Autodesk Inventor part; units mm, degrees
ref_plane "YZ Plane" through (0, 0, 0) normal (1, 0, 0) x (0, 1, 0)
ref_plane "XZ Plane" through (0, 0, 0) normal (0, 1, 0) x (-1, 0, 0)
ref_plane "XY Plane" through (0, 0, 0) normal (0, 0, 1) x (1, 0, 0)
sketch "Sketch15" plane through (0, 0, 0) normal (0, 0, 1) x (1, 0, 0)
  line L0 (0, 0) -> (0, 1.4)
  line L1 (0.2309, 1.8) -> (1.5, 1.8)
  line L2 (1.5, 1.8) -> (1.5, 2)
  line L3 (1.5, 2) -> (1.7, 2)
  line L4 (1.7, 2) -> (1.7, 1)
  line L5 (1.7, 1) -> (5.7, 1)
  line L6 (5.7, 0) -> (0, 0)
  line L7 (0.2309, 1.8) -> (0, 1.4)
  line L8 (5.7, 1) -> (5.7, 0)
  point P0 (6.0083, 0)
  dimension "d78" = 0.2
  dimension "d84" = 1
  dimension "d86" = 0.4
  dimension "d87" = 1.8
  dimension "d89" = 1.5
  dimension "d90" = 2
  dimension "d111" = 4
revolve "Revolution1" add sketch "Sketch15" angle 360 about axis through (5.7, 0, 0) along (-1, 0, 0)
chamfer "Chamfer4" distance 0.2 angle 45 1 edges at (5.7, -1, 0)
sketch "Sketch16" plane through (0, 0, 0) normal (-1, 0, 0) x (0, 0, 1)
  circle A0 centre (0, 0) radius 1.4
  line L0 (0.9238, 1.6) -> (1.8475, 0)
  line L1 (1.8475, 0) -> (0.9238, -1.6)
  line L2 (0.9238, -1.6) -> (-0.9238, -1.6)
  line L3 (-0.9238, -1.6) -> (-1.8475, 0)
  line L4 (-1.8475, 0) -> (-0.9238, 1.6)
  line L5 (-0.9238, 1.6) -> (0.9238, 1.6)
  circle A1 centre (0, 0) radius 2.6573
  dimension "d104" = 3.2
extrude "Extrusion15" cut sketch "Sketch16" against normal up to surface (1.5 mm away) contours A1
thread "Thread3"
properties part number "Bolt2b"
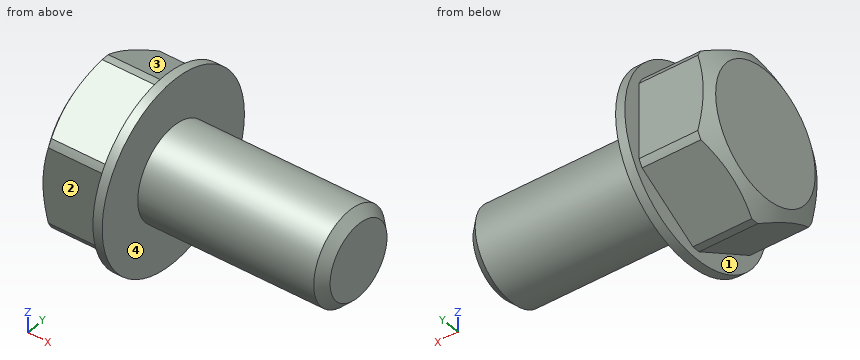
Design review of the part built by this model. Coordinates are the model's own, in mm. Face numbers are marked on the shaded views. A direction names the side the tool comes from. Coordinates: 2 decimals unless noted, no trailing zeros. Order: outer loops, then holes, each group sorted by start corner. A loop starts at its lowest first (then second) coordinate and runs counter-clockwise, first axis right, second up. Notation, with made-up numbers: (17, 5) -> (72, 5) arc R32 cw to (72, 44) -> close; hole circle Ø4 at (87, -2.5). An arc over 180 degrees is marked (long way). One line per item, written item: value. Start each with the question number.
Q1. Take a section at B-B, the plane z = 0. State the section outline as (x, y) points.
Q2. Take a section at A-A, the plane y = 0. State the section outline as (x, z) points.
Q3. Insertion check: pin 1 Ø1 at (x, z) = (3.5, 0.5) entering from -Y; pin 2 Ø1.1 at (x, z) = (0.5, -0.5) entering from -Y; pin 3 Ø0.7 at (x, z) = (1, 0.5) entering from +Y. Each pin has a flat end and moves straight along its axis. Give the tip position at first contact, or say it passes through.
Q4. For probe 1 along X at (y, z) = (-1.15, -0.6); probe 2 along Z at (x, y) = (4.45, -0.05); probe 3 along Y at (x, z) = (0.4, -0.05), list the stretches that pass through material, from the lowest coordinate up.
Q5. Tool access review of the marked faces 1, 2, 3 and 4: name each direction out of +Z, -Z, +X, -X, +Y, -Y from which nothing blocks a thin tool from reaching the whole face with its end or side.
Q6. Take a section at C-C, the plane x = 2.5. State the section outline as (y, z) points, then the cut area to 3 significant figures.
Values follow:
1. outline: (0, -1.4) -> (0.12, -1.6) -> (1.5, -1.6) -> (1.5, -2) -> (1.7, -2) -> (1.7, -1) -> (5.5, -1) -> (5.7, -0.8) -> (5.7, 0.8) -> (5.5, 1) -> (1.7, 1) -> (1.7, 2) -> (1.5, 2) -> (1.5, 1.6) -> (0.12, 1.6) -> (0, 1.4) -> close
2. outline: (0, -1.4) -> (0.23, -1.8) -> (1.5, -1.8) -> (1.5, -2) -> (1.7, -2) -> (1.7, -1) -> (5.5, -1) -> (5.7, -0.8) -> (5.7, 0.8) -> (5.5, 1) -> (1.7, 1) -> (1.7, 2) -> (1.5, 2) -> (1.5, 1.8) -> (0.23, 1.8) -> (0, 1.4) -> close
3. pin 1: stops at y = -1
3. pin 2: stops at y = -1.6
3. pin 3: stops at y = 1.6
4. probe 1: x = 0 to 1.7
4. probe 2: z = -1 to 1
4. probe 3: y = -1.6 to 1.6
5. face 1: -X
5. face 2: +Z, -Z, -X, -Y
5. face 3: +Z, -X, +Y
5. face 4: +X
6. outline: circle Ø2 at (0, 0)
6. area: 3.14 mm2
